Check sheet for the modelled part. Datum: model origin and axes. Units: mm. A direction names the side the tool comes from. Give positions to 0.01 mm unless a question says otherwise; leave off trailing zeros. Loops run counter-clockwise (first coordinate to the right, second up) from the corner with the lowest first, then second, coordinate; pieces in that order, holes last. Notation, with made-up numbers: (24.5, 21) - (60.5, 21) arc R17 cw to (60.5, 42) - close; hole circle Ø9 at (18, 3.5). An arc over 180 degrees is marked (long way). Answer in a Markdown table with one row per item. Add a question column.
(1) Thickness scan on L1, parallel to Z at x = 19.5, y = 15.5; L2, parallel to Y at x = -30.5, z = 5.5; L3, parallel to Z at x = -4, y = 16. Record the ranges inside material, lowest first.
(2) Sectioned sample at D-D on x = -25.5. Enter the section's corners in (y, z).
(3) Sectioned sample at C-C on y = 19. Enter the section's corners in (x, z).
(4) Sectioned sample at B-B on x = -2. Enter the section's corners in (y, z), then the cut area to 3 significant figures.
(5) Sectioned sample at A-A on z = 3.25. Enter the section's corners in (x, y), then the cut area to 3 significant figures.
(6) Set-up check for faces 1 (the face through (-5, 0, 0)), 2 (the face through (-8.229, 17.968, 4.418)): record each of +Z, -Z, +X, -X, +Y, -Y from which the full face is reachable in a straight line by a thin tool's end or side.
(7) Draft check along X on faces 3 (the face through (-8.76, 20.5, 3.13)), 4 (the face through (-32.91, 0.32, 4.42)), 5 (the face through (25.923, -0.57, 3.131)). Enter one of: released by +X, released by -X, zero draft, split by the parting line, or undercut.
(8) Go/stop test with flat-tipped pins: P1, Ø2, axis at x = 16, z = 8, coming from the +Y side; P2, Ø1.5, axis at x = 14, z = 2.5, coming from the +Y side; P3, Ø4, axis at y = -5, z = 5.5, coming from the -X side; P4, Ø6, axis at x = -0.5, y = -10.5, coming from the +Z side. Record where each tip stops, or that it passes through.
from build123d import *

# Parameters (mm, degrees)
BOSS_EXTRUDE1_DEPTH = 6.35
SHELL1_T            = -2.54
SKETCH2_R           = 0.508
BOSS_EXTRUDE2_DEPTH = 3.81
SKETCH3_R           = 4.826
SKETCH3_R_2         = 3.175
CUT_EXTRUDE1_DEPTH  = 2.54


with BuildPart() as part:
    # Sketch1 → Boss-Extrude1 (new body)
    with BuildSketch(Plane.XY):
        with BuildLine():
            ThreePointArc((0, -25.92959), (25.92959, 0), (0, 25.92959))
            ThreePointArc((0, 25.92959), (-8.900253562, 20.439501874), (-19.05, 17.921918042))
            ThreePointArc((-19.05, 17.921918042), (-35.45459, 0), (-19.05, -17.921918042))
            ThreePointArc((-19.05, -17.921918042), (-8.900253562, -20.439501874), (0, -25.92959))
        make_face()
    extrude(amount=BOSS_EXTRUDE1_DEPTH)

    # Shell1
    shell1_openings = [part.faces().sort_by_distance(p)[0] for p in [
        (-3.11409352, 0, 6.35),
    ]]
    offset(amount=SHELL1_T, openings=shell1_openings, kind=Kind.INTERSECTION)

    # Sketch2 → Boss-Extrude2 (add)
    with BuildSketch(Plane.XY.offset(6.35)):
        with Locations((-34.39268404, 0)):
            Circle(SKETCH2_R)
        with Locations((24.569143143, 0)):
            Circle(SKETCH2_R)
    extrude(amount=BOSS_EXTRUDE2_DEPTH)

    # Sketch3 → Cut-Extrude1 (cut)
    with BuildSketch(Plane.XY.offset(2.54)):
        Circle(SKETCH3_R)
        with Locations((-17.4625, 0)):
            Circle(SKETCH3_R_2)
    extrude(amount=-CUT_EXTRUDE1_DEPTH, mode=Mode.SUBTRACT)


solid = part.part
Reply:
| question | item | result |
|---|---|---|
| 1 | L1 | 0 to 6.35 |
| 1 | L2 | -12.4 to -8.29, 8.29 to 12.4 |
| 1 | L3 | 0 to 2.54 |
| 2 | outline | (-16.1, 0) - (16.1, 0) - (16.1, 6.35) - (13.2, 6.35) - (13.2, 2.54) - (-13.2, 2.54) - (-13.2, 6.35) - (-16.1, 6.35) - close |
| 3 | outline | (-13.06, 0) - (17.64, 0) - (17.64, 6.35) - (13.64, 6.35) - (13.64, 2.54) - (-5.94, 2.54) - (-5.94, 6.35) - (-13.06, 6.35) - close |
| 4 | outline | (-24.35, 0) - (-4.39, 0) - (-4.39, 2.54) - (-21.25, 2.54) - (-21.25, 6.35) - (-24.35, 6.35) - close; (4.39, 0) - (24.35, 0) - (24.35, 6.35) - (21.25, 6.35) - (21.25, 2.54) - (4.39, 2.54) - close |
| 4 | area | 125 mm^2 |
| 5 | outline | (-19.05, -17.92) arc R33.91 cw to (0, -25.93) arc R25.93 ccw to (0, 25.93) arc R33.91 cw to (-19.05, 17.92) arc R17.99 ccw to start; hole (-18.83, -15.39) arc R36.45 cw to (0.9, -23.37) arc R23.39 ccw to (0.9, 23.37) arc R36.45 cw to (-18.83, 15.39) arc R15.45 ccw to start |
| 5 | area | 429 mm^2 |
| 6 | face 1 | -Z, +X, -X, +Y, -Y |
| 6 | face 2 | +Z |
| 7 | face 3 | released by -X |
| 7 | face 4 | undercut |
| 7 | face 5 | released by +X |
| 8 | P1 | through |
| 8 | P2 | y = 22.29 |
| 8 | P3 | x = -35.2 |
| 8 | P4 | z = 2.54 |
